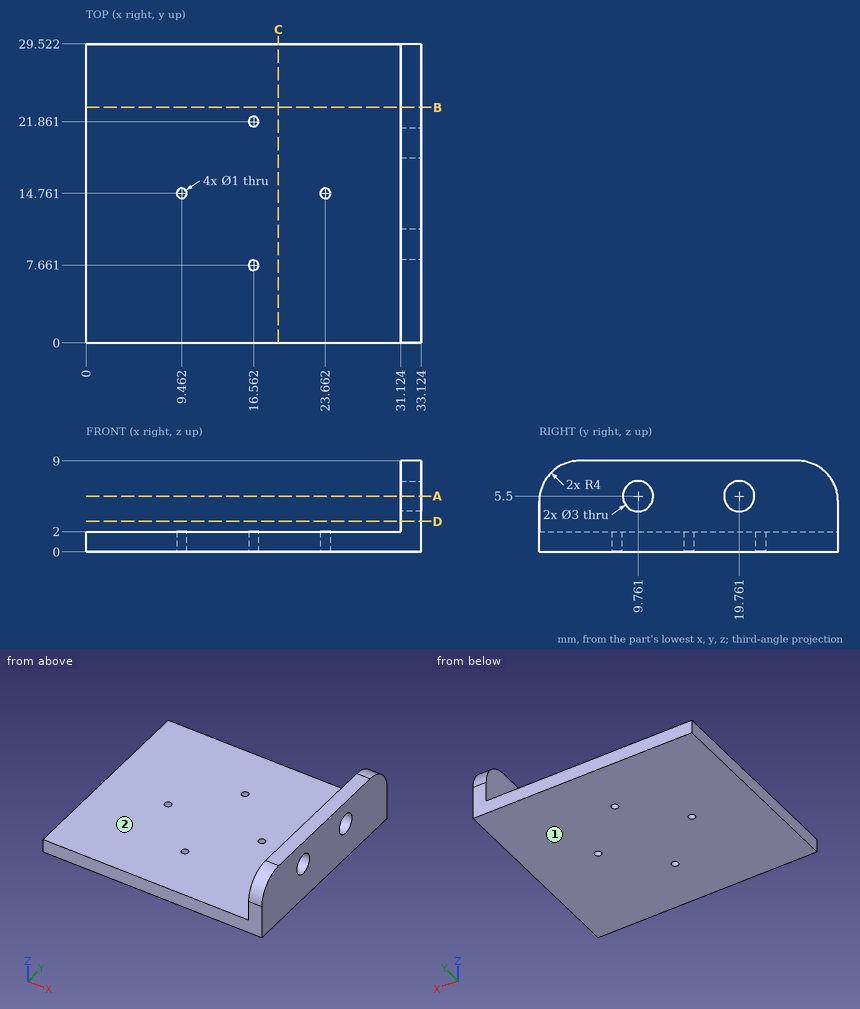
Print and shaded views of the part. All mm, measured from the part's lowest x, y and z. A direction names the side the tool comes from. Give positions to 0.01 mm unless a question says otherwise; leave off trailing zeros. Loops run counter-clockwise (first coordinate to the right, second up) from the corner with the lowest first, then second, coordinate; pieces in that order, holes last. Notation, with made-up numbers: (-13.75, 63) -> (21.25, 63) arc R25 cw to (21.25, 87) -> close; hole circle Ø4 at (25.25, -30). An arc over 180 degrees is marked (long way). One line per question, with ' | ' between items. Start each with the question number.
1) Cut at B-B (y = 23.25). Give the cut face in (x, z).
2) Cut at D-D (z = 3). Give the cut face in (x, y).
3) Pin check, flat tips, straight feed: pin 1 (6 mm diameter, centred on x = 13.5, y = 25.5, fed in from -Z); pin 2 (2 mm diameter, centred on x = 23.5, z = 4, fed in from +Y); pin 3 (4 mm diameter, centred on x = 10, y = 14.5, fed in from +Z). Stop position of each tip, or through.
4) Cut at A-A (z = 5.5). Give the cut face in (x, y), plus the area to 3 significant figures.
5) 3-axis set-ups, long thin cutter, end or side, ignore diameter. For the marked faces 1 and 2: which of +Z, -Z, +X, -X, +Y, -Y reach the whole face in a straight line?
6) Probe L1, parallel to Y at x = 32.5, z = 5.5; L2, parallel to Z at x = 20.5, y = 13; L3, parallel to X at y = 4.5, z = 8.25. List the from-to ranges inside material, lowest first.
7) Cut at C-C (x = 19). Give the cut face in (y, z).
Return value:
1) outline: (0, 0) -> (33.12, 0) -> (33.12, 9) -> (31.12, 9) -> (31.12, 2) -> (0, 2) -> close
2) outline: (31.12, 0) -> (33.12, 0) -> (33.12, 29.52) -> (31.12, 29.52) -> close
3) pin 1: z = 0 | pin 2: through | pin 3: z = 2
4) outline: (31.12, 0.03) -> (33.12, 0.03) -> (33.12, 8.26) -> (31.12, 8.26) -> close; (31.12, 11.26) -> (33.12, 11.26) -> (33.12, 18.26) -> (31.12, 18.26) -> close; (31.12, 21.26) -> (33.12, 21.26) -> (33.12, 29.49) -> (31.12, 29.49) -> close | area: 46.9 mm^2
5) face 1: -Z, +X, -X, +Y, -Y | face 2: +Z, -X, +Y, -Y
6) L1: 0.03 to 8.26, 11.26 to 18.26, 21.26 to 29.49 | L2: 0 to 2 | L3: 31.12 to 33.12
7) outline: (0, 0) -> (29.52, 0) -> (29.52, 2) -> (0, 2) -> close
